For this review, take the finished solid that the model builds, in its own axes (mm). Face numbers are marked on the shaded views. A direction names the side the tool comes from. Coordinates: 2 decimals unless noted, no trailing zeros. Loops run counter-clockwise (first coordinate to the right, second up) from the corner with the lowest first, then second, coordinate; pieces in that order, holes last.
```python
from build123d import *

# Parameters (mm, degrees)
EXTRUDE_1_DEPTH     = 100
CUT_EXTRUDE_1_DEPTH = 10
SKETCH_3_R          = 1.75
CUT_EXTRUDE_2_DEPTH = 10
SKETCH_4_R          = 1.75
CUT_EXTRUDE_3_DEPTH = 10


with BuildPart() as part:
    # Эскиз1 → Бобышка-Вытянуть1 (new body)
    with BuildSketch(Plane(origin=(0, 0, 0), x_dir=(1, 0, 0), z_dir=(0, 1, 0))):
        with BuildLine():
            Line((0, 0), (-112.5, 0))
            ThreePointArc((-112.5, 0), (-119.571067812, -2.928932188), (-122.5, -10))
            Line((-122.5, -10), (-122.5, -50))
            ThreePointArc((-122.5, -50), (-123.964466094, -53.535533906), (-127.5, -55))
            Line((-127.5, -55), (-127.5, -53))
            Line((-127.5, -53), (-137.5, -53))
            Line((-137.5, -53), (-137.5, -51.5))
            Line((-137.5, -51.5), (-124, -51.5))
            Line((-124, -51.5), (-124, 1.5))
            Line((-124, 1.5), (1.5, 1.5))
            Line((1.5, 1.5), (1.5, 15))
            Line((1.5, 15), (3, 15))
            Line((3, 15), (3, 5))
            Line((3, 5), (5, 5))
            ThreePointArc((5, 5), (3.535533906, 1.464466094), (0, 0))
        make_face()
    extrude(amount=EXTRUDE_1_DEPTH)

    # Эскиз2 → Вырез-Вытянуть1 (cut)
    with BuildSketch(Plane.XY):
        with BuildLine():
            Line((-73, 100), (-37, 100))
            Line((-37, 100), (-37, 82.000001723))
            ThreePointArc((-37, 82.000001723), (-54.999999139, 64.000000861), (-73, 82))
            Line((-73, 82), (-73, 100))
        make_face()
    extrude(amount=-CUT_EXTRUDE_1_DEPTH, mode=Mode.SUBTRACT)

    # Эскиз3 → Вырез-Вытянуть2 (cut)
    with BuildSketch(Plane(origin=(3, 0, 0), x_dir=(0, 0, -1), z_dir=(1, 0, 0))):
        with Locations((10, 90)):
            Circle(SKETCH_3_R)
        with Locations((10, 10)):
            Circle(SKETCH_3_R)
    extrude(amount=-CUT_EXTRUDE_2_DEPTH, mode=Mode.SUBTRACT)

    # Эскиз4 → Вырез-Вытянуть3 (cut)
    with BuildSketch(Plane.XY.offset(53)):
        with Locations((-132.5, 90)):
            Circle(SKETCH_4_R)
        with Locations((-132.5, 10)):
            Circle(SKETCH_4_R)
    extrude(amount=-CUT_EXTRUDE_3_DEPTH, mode=Mode.SUBTRACT)


solid = part.part
```
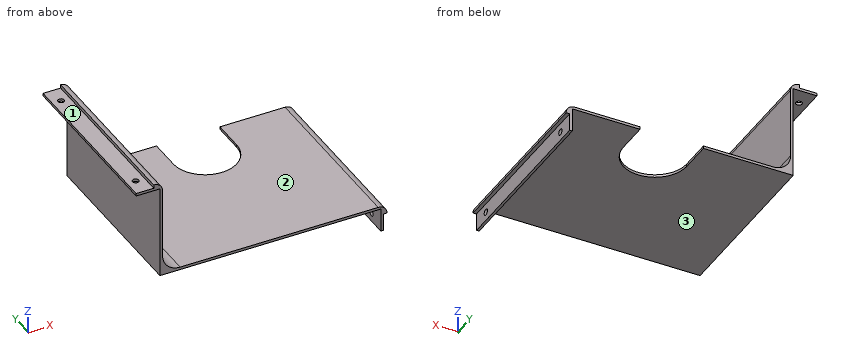
Q1. Consider section C-C (x = -132.5). State the section outline as (y, z) points, then the cut area to 4 significant figures.
Q2. For pin 1 Ø1.5 at (y, z) = (44, 13.5) entering from +X; pin 2 Ø1.6 at (y, z) = (93, -1) entering from -X; pin 3 Ø6 at (x, y) = (-17, 27) entering from -Z, all flat-tipped, find the tip position at first contact; note any pin that passes through.
Q3. Consider section B-B (y = 10). State the section outline as (x, z) points.
Q4. Consider section D-D (y = 67.5). State the section outline as (x, z) points.
Q5. Consider section A-A (z = -10). State the section outline as (x, y) points, then the cut area to 4 significant figures.
Q6. Machinability: for the marked faces 1, 2 and 3, which of the approach directions +Z, -Z, +X, -X, +Y, -Y give a long, thin tool a straight path to every point of the face, cutting with its end or side? Answer none if there is none.
Q7. Wall thickness on probe 1 along Y at (x, z) = (-132.5, 52.6); probe 2 along Z at (x, y) = (-18, 44); probe 3 along X at (y, z) = (63.5, 44): over which ranges is each line inside the solid? List them lowest first.
Model answer:
1. outline: (0, 51.5) - (8.25, 51.5) - (8.25, 53) - (0, 53) - close; (11.75, 51.5) - (88.25, 51.5) - (88.25, 53) - (11.75, 53) - close; (91.75, 51.5) - (100, 51.5) - (100, 53) - (91.75, 53) - close
1. area: 139.5 mm2
2. pin 1: stops at x = -122.5
2. pin 2: stops at x = -124
2. pin 3: stops at z = -1.5
3. outline: (-137.5, 51.5) - (-134.25, 51.5) - (-134.25, 53) - (-137.5, 53) - close; (-130.75, 51.5) - (-124, 51.5) - (-124, -1.5) - (1.5, -1.5) - (1.5, -8.25) - (3, -8.25) - (3, -5) - (5, -5) arc R5 ccw to (0, 0) - (-112.5, 0) arc R10 cw to (-122.5, 10) - (-122.5, 50) arc R5 ccw to (-127.5, 55) - (-127.5, 53) - (-130.75, 53) - close; (1.5, -15) - (3, -15) - (3, -11.75) - (1.5, -11.75) - close
4. outline: (-137.5, 51.5) - (-124, 51.5) - (-124, -1.5) - (-65.67, -1.5) - (-65.67, 0) - (-112.5, 0) arc R10 cw to (-122.5, 10) - (-122.5, 50) arc R5 ccw to (-127.5, 55) - (-127.5, 53) - (-137.5, 53) - close; (-44.33, -1.5) - (1.5, -1.5) - (1.5, -15) - (3, -15) - (3, -5) - (5, -5) arc R5 ccw to (0, 0) - (-44.33, 0) - close
5. outline: (1.5, 0) - (3, 0) - (3, 8.25) - (1.5, 8.25) - close; (1.5, 11.75) - (3, 11.75) - (3, 88.25) - (1.5, 88.25) - close; (1.5, 91.75) - (3, 91.75) - (3, 100) - (1.5, 100) - close
5. area: 139.5 mm2
6. face 1: +Z, -X, +Y, -Y
6. face 2: +Z, +X, +Y, -Y
6. face 3: -Z, -X, +Y, -Y
7. probe 1: y = 0 to 8.25, 11.75 to 88.25, 91.75 to 100
7. probe 2: z = -1.5 to 0
7. probe 3: x = -124 to -122.5
